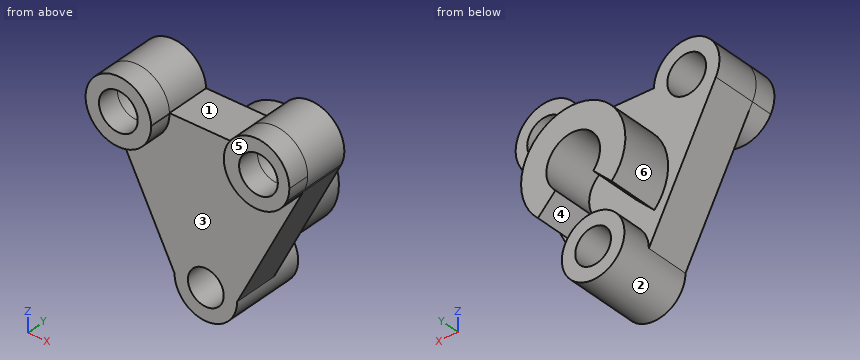
```python
from build123d import *

# Parameters (mm, degrees)
SKETCH2_R           = 13
BOSS_EXTRUDE1_DEPTH = 30
SKETCH3_R           = 21
SKETCH3_R_2         = 12
BOSS_EXTRUDE3_DEPTH = 30
BOSS_EXTRUDE4_START = 20
SKETCH4_R           = 21
BOSS_EXTRUDE4_DEPTH = 20
CUT_EXTRUDE3_START  = 20
SKETCH6_R           = 12
CUT_EXTRUDE3_DEPTH  = 20
BOSS_EXTRUDE5_DEPTH = 35
SKETCH8_R           = 13
BOSS_EXTRUDE6_DEPTH = 15


with BuildPart() as part:
    # Sketch2 → Boss-Extrude1 (new body)
    with BuildSketch(Plane(origin=(0, 0, 0), x_dir=(1, 0, 0), z_dir=(0, 1, 0))):
        with BuildLine():
            Line((-63.748151168, 83.4945297), (-108.720702631, -4.492807031))
            ThreePointArc((-108.720702631, -4.492807031), (-94.582688401, -35.819358768), (-67.140057524, -15.127855665))
            Line((-67.140057524, -15.127855665), (-18.356244812, -15.127855665))
            ThreePointArc((-18.356244812, -15.127855665), (8.155744942, -36.660202227), (23.79302323, -6.295698659))
            Line((23.79302323, -6.295698659), (22.673576153, -4.088566102))
            Line((22.673576153, -4.088566102), (-21.748151168, 83.4945297))
            ThreePointArc((-21.748151168, 83.4945297), (-42.748151168, 62.4945297), (-63.748151168, 83.4945297))
        make_face()
        with Locations(Location((-89.131252045, -14.5054703, 0), (0, 0, 270))):
            Circle(SKETCH2_R, mode=Mode.SUBTRACT)
        with Locations(Location((4.884095697, -15.127855665, 0), (0, 0, 270))):
            Circle(SKETCH2_R, mode=Mode.SUBTRACT)
    extrude(amount=-BOSS_EXTRUDE1_DEPTH)

    # Sketch3 → Boss-Extrude3 (add)
    with BuildSketch(Plane(origin=(0, 0, 0), x_dir=(1, 0, 0), z_dir=(0, 1, 0))):
        with Locations((-42.748151168, 83.4945297)):
            Circle(SKETCH3_R)
        with Locations(Location((-42.748151168, 83.4945297, 0), (0, 0, 270))):
            Circle(SKETCH3_R_2, mode=Mode.SUBTRACT)
    extrude(amount=-BOSS_EXTRUDE3_DEPTH)

    # Sketch4 → Boss-Extrude4 (add)
    with BuildSketch(Plane(origin=(0, 0, 0), x_dir=(1, 0, 0), z_dir=(0, 1, 0)).offset(BOSS_EXTRUDE4_START)):
        with Locations(Location((-42.748151168, 83.4945297, 0), (0, 0, 270))):
            Circle(SKETCH4_R)
    extrude(amount=-BOSS_EXTRUDE4_DEPTH)

    # Sketch6 → Cut-Extrude3 (cut)
    with BuildSketch(Plane(origin=(0, 0, 0), x_dir=(1, 0, 0), z_dir=(0, 1, 0)).offset(CUT_EXTRUDE3_START)):
        with Locations(Location((-42.748151168, 83.4945297, 0), (0, 0, 270))):
            Circle(SKETCH6_R)
    extrude(amount=-CUT_EXTRUDE3_DEPTH, mode=Mode.SUBTRACT)

    # Sketch7 → Boss-Extrude5 (add)
    with BuildSketch(Plane(origin=(0, 0, 0), x_dir=(1, 0, 0), z_dir=(0, 1, 0))):
        with BuildLine():
            Line((-55.137118112, 49.462443333), (-67.471148686, 61.168135895))
            ThreePointArc((-67.471148686, 61.168135895), (-40.20329361, 2.526208117), (-18.018474049, 63.273598143))
            Line((-18.018474049, 63.273598143), (-29.724166611, 50.939567569))
            ThreePointArc((-29.724166611, 50.939567569), (-40.647595679, 19.524859364), (-55.137118112, 49.462443333))
        make_face()
    extrude(amount=BOSS_EXTRUDE5_DEPTH)

    # Sketch8 → Boss-Extrude6 (add)
    # profile 1 of 2: a face of its own
    with BuildSketch(Plane.XZ.offset(30)):
        with BuildLine():
            ThreePointArc((25.643755188, 15.127855665), (3.643755188, 37.127855665), (-18.356244812, 15.127855665))
            ThreePointArc((-18.356244812, 15.127855665), (-2.072184751, -6.116626692), (22.673576153, 4.088566102))
            Line((22.673576153, 4.088566102), (23.79302323, 6.295698659))
            ThreePointArc((23.79302323, 6.295698659), (25.17610175, 10.615865911), (25.643755188, 15.127855665))
        make_face()
        with Locations(Location((4.884095697, 15.127855665, 0), (0, 0, 90))):
            Circle(SKETCH8_R, mode=Mode.SUBTRACT)
    # profile 2 of 2: a face of its own
    with BuildSketch(Plane.XZ.offset(30)):
        with BuildLine():
            ThreePointArc((-67.131252045, 14.5054703), (-67.133453525, 14.816694125), (-67.140057524, 15.127855665))
            ThreePointArc((-67.140057524, 15.127855665), (-94.582688401, 35.819358768), (-108.720702631, 4.492807031))
            ThreePointArc((-108.720702631, 4.492807031), (-83.981878922, -6.883404296), (-67.131252045, 14.5054703))
        make_face()
        with Locations(Location((-89.131252045, 14.5054703, 0), (0, 0, 90))):
            Circle(SKETCH8_R, mode=Mode.SUBTRACT)
    extrude(amount=BOSS_EXTRUDE6_DEPTH)


solid = part.part
```
Model file for the job. Use its own axes, mm. Face numbers are marked on the shaded views. A direction names the side the tool comes from. Coordinates: 2 decimals unless noted, no trailing zeros. Loops run counter-clockwise (first coordinate to the right, second up) from the corner with the lowest first, then second, coordinate; pieces in that order, holes last. Notation, with made-up numbers: (60, 56) -> (72, 56) arc R22 ccw to (72, 73) -> close; hole circle Ø2 at (11.25, -20.5). An arc over 180 degrees is marked (long way). Answer as a JSON object with one key per item and string values.
Q1. Cut at A-A (y = -37). List the corners of the cut face in (x, z), and give its area (3 significant figures).
Report:
{"outline": "(-67.14, 15.13) arc R22 ccw (long way) to (-67.13, 14.51) arc R22 ccw to start; (22.67, 4.09) -> (23.79, 6.3) arc R22 ccw (long way) to start; hole circle Ø26 at (-89.13, 14.51); hole circle Ø26 at (4.88, 15.13)", "area": "1,980 mm2"}
Q2. 3-axis set-ups, long thin cutter, end or side, ignore diameter. For the marked faces 1, 2 and 3: which of +Z, -Z, +X, -X, +Y, -Y reach the whole face in a straight line?
Report:
{"face 1": "+Z, +Y, -Y", "face 2": "+Y", "face 3": "-Z, -Y"}
Q3. Cut at B-B (z = -91). List the corners of the cut face in (x, y), and give its area (3 significant figures).
Report:
{"outline": "(-62.36, -30) -> (-52.11, -30) -> (-52.11, 20) -> (-62.36, 20) -> close; (-33.39, -30) -> (-23.14, -30) -> (-23.14, 20) -> (-33.39, 20) -> close", "area": "1,020 mm2"}
Q4. Flat gauge pins, fed straight in: P1, Ø5, axis at y = 1.5, z = 6, coming from the -X side; P2, Ø5, axis at x = -53, y = -18.5, coming from the +Z side; P3, Ø10, axis at y = 7.5, z = -25.5, coming from the -X side. Where does each tip first touch, or does it go through?
Report:
{"P1": "stops at x = -110.15", "P2": "stops at z = 15.13", "P3": "stops at x = -75.99"}
Q5. Probe probe 1 along Z at (x, y) = (-47.5, 4.5); probe 2 along X at (y, z) = (-3.5, -80); probe 3 along Y at (x, z) = (-73, -51.5). List the from-to ranges inside material, lowest first.
Report:
{"probe 1": "z = -103.95 to -94.51, -72.48 to -63.04, -20.46 to -2.98", "probe 2": "x = -65.53 to -54.23, -31.27 to -19.98", "probe 3": "y = -30 to 35"}
Q6. Cut at D-D (y = 8). List the corners of the cut face in (x, z).
Report:
{"outline": "(-67.47, -61.17) -> (-55.14, -49.46) arc R18 cw (long way) to (-29.72, -50.94) -> (-18.02, -63.27) arc R35 ccw (long way) to start; circle Ø42 at (-42.75, -83.49); hole circle Ø24 at (-42.75, -83.49)"}
Q7. Pull direction X, two halves, no side cores. Call the marked faces 4, 5 and 6: released by +X, released by -X, zero draft, split by the parting line, or undercut.
Report:
{"face 4": "undercut", "face 5": "zero draft", "face 6": "split by the parting line"}
Q8. Cut at C-C (x = -95.5). List the corners of the cut face in (y, z).
Report:
{"outline": "(-45, -6.55) -> (-30, -6.55) -> (-30, -21.37) -> (0, -21.37) -> (0, 3.17) -> (-45, 3.17) -> close; (-45, 25.84) -> (0, 25.84) -> (0, 35.56) -> (-45, 35.56) -> close"}
